```python
from build123d import *

# Parameters (mm, degrees)
SKETCH1_R               = 21
SKETCH1_R_2             = 16
BOSS_EXTRUDE1_DEPTH     = 10
SKETCH1_R_3             = 12.5
SKETCH1_R_4             = 6.25
BOSS_EXTRUDE1_2_DEPTH   = 10
BOSS_EXTRUDE2_DEPTH     = 6
CUT_EXTRUDE1_START      = -6
CUT_EXTRUDE1_DEPTH      = 22
CUT_EXTRUDE1_DEPTH_BACK = 16


with BuildPart() as part:
    # Sketch1 → Boss-Extrude1 (new body, symmetric)
    with BuildSketch(Plane.XY):
        Circle(SKETCH1_R)
        Circle(SKETCH1_R_2, mode=Mode.SUBTRACT)
    extrude(amount=BOSS_EXTRUDE1_DEPTH, both=True)



with BuildPart() as body_2:
    # Sketch1 → Boss-Extrude1 2 (new body, symmetric)
    with BuildSketch(Plane.XY):
        with Locations((0, 120)):
            Circle(SKETCH1_R_3)
        with Locations((0, 120)):
            Circle(SKETCH1_R_4, mode=Mode.SUBTRACT)
    extrude(amount=BOSS_EXTRUDE1_2_DEPTH, both=True)


with BuildPart() as part_1:
    add(part.part)

    add(body_2.part)  # Boss-Extrude2 merges body 2
    # Sketch1<4> → Boss-Extrude2 (add, symmetric)
    with BuildSketch(Plane.XY):
        with BuildLine():
            Line((-8, 110.395313644), (-8, 75.395313644))
            ThreePointArc((-8, 75.395313644), (-10.96842855, 40.709642053), (-19.787382488, 7.032744434))
            ThreePointArc((-19.787382488, 7.032744434), (0, 21), (19.787382488, 7.032744434))
            ThreePointArc((19.787382488, 7.032744434), (10.96842855, 40.709642053), (8, 75.395313644))
            Line((8, 75.395313644), (8, 110.395313644))
            ThreePointArc((8, 110.395313644), (0, 107.5), (-8, 110.395313644))
        make_face()
        with BuildLine():
            Line((-6.25, 135.825317547), (-6.25, 130.825317547))
            ThreePointArc((-6.25, 130.825317547), (0, 132.5), (6.25, 130.825317547))
            Line((6.25, 130.825317547), (6.25, 135.825317547))
            Line((6.25, 135.825317547), (-6.25, 135.825317547))
        make_face()
        with BuildLine():
            ThreePointArc((17, -12.328828006), (0, -21), (-17, -12.328828006))
            Line((-17, -12.328828006), (-17, -24.328828006))
            Line((-17, -24.328828006), (17, -24.328828006))
            Line((17, -24.328828006), (17, -12.328828006))
        make_face()
    extrude(amount=BOSS_EXTRUDE2_DEPTH, both=True)

    # Sketch2 → Cut-Extrude1 (cut, two sides)
    with BuildSketch(Plane(origin=(0, 0, 0), x_dir=(0, 0, -1), z_dir=(1, 0, 0)).offset(CUT_EXTRUDE1_START)) as cut_extrude1_sk:
        with BuildLine():
            Line((4, 100), (4, 38))
            ThreePointArc((4, 38), (0, 34), (-4, 38))
            Line((-4, 38), (-4, 100))
            ThreePointArc((-4, 100), (0, 104), (4, 100))
        make_face()
    extrude(amount=CUT_EXTRUDE1_DEPTH, mode=Mode.SUBTRACT)
    extrude(cut_extrude1_sk.sketch, amount=-CUT_EXTRUDE1_DEPTH_BACK, mode=Mode.SUBTRACT)


solid = part_1.part
```
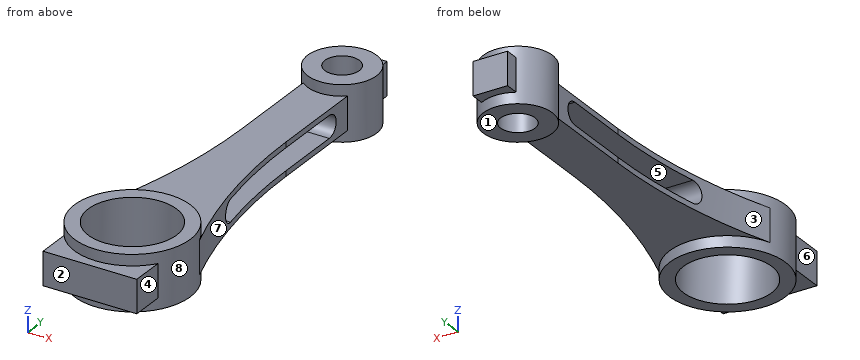
Input: part model. Units: mm. Frame: model coordinates. Face numbers are marked on the shaded views. A direction names the side the tool comes from. Round coordinates to 2 decimals unless told otherwise and drop trailing zeros. Write each loop counter-clockwise with the first axis right and the second up, starting at its lowest first coordinate (ties: lowest second). Pieces come first, ordered by that corner, then holes. Notation, with made-up numbers: (9, -30) - (59, -30) arc R14 ccw to (59, -15) - close; hole circle Ø10 at (85.5, 19). An arc over 180 degrees is marked (long way). Write item = value, one per line.
(1) Pull-direction query (Y, two-part tool) for the marked faces 1, 2 and 3; classes: +Y half, -Y half, draft (parallel to the pull), parting line (faces both ways), or undercut.
Geometry check:
face_1 = draft
face_2 = -Y half
face_3 = undercut
(2) Section query D-D on y = 120. Output: boundary loops of the cut face in (x, z), then the cut area to 3 significant figures.
Geometry check:
outline = (-12.5, -10) - (-6.25, -10) - (-6.25, 10) - (-12.5, 10) - close; (6.25, -10) - (12.5, -10) - (12.5, 10) - (6.25, 10) - close
area = 250 mm^2
(3) Section query C-C on y = 86.5. Output: boundary loops of the cut face in (x, z), then the cut area to 3 significant figures.
Geometry check:
outline = (-8, -6) - (8, -6) - (8, -4) - (-8, -4) - close; (-8, 4) - (8, 4) - (8, 6) - (-8, 6) - close
area = 64.0 mm^2
(4) Contact query for flat-ended pins moving along their axis: pin 1 Ø10 at (x, y) = (6, 94) entering from +Z; pin 2 Ø1 at (x, z) = (11.5, 5.5) entering from +Y; pin 3 Ø25 at (x, y) = (-2, 66) entering from -Z. Output: stop coordinate, or through.
Geometry check:
pin_1 = 6
pin_2 = 125.94
pin_3 = -6
(5) Section query B-B on z = 0. Output: boundary loops of the cut face in (x, y).
Geometry check:
outline = (-19.79, 7.03) arc R21 ccw to (-17, -12.33) - (-17, -24.33) - (17, -24.33) - (17, -12.33) arc R21 ccw to (19.79, 7.03) arc R204.13 cw to (12.24, 34) - (-12.24, 34) arc R204.13 cw to start; (-8, 104) - (8, 104) - (8, 110.4) arc R12.5 ccw to (6.25, 130.83) - (6.25, 135.83) - (-6.25, 135.83) - (-6.25, 130.83) arc R12.5 ccw to (-8, 110.4) - close; hole circle Ø32 at (0, 0); hole circle Ø12.5 at (0, 120)
(6) Section query A-A on x = 0. State how many separate pieces and enclosed holes the cut face has, then the cut area to 3 significant figures.
Geometry check:
separate_pieces = 3
enclosed_holes = 1
area = 1,020 mm^2
(7) Access query for the marked faces 4, 5, 6, 7 and 8. Directions: +Z, -Z, +X, -X, +Y, -Y. A direction counts if a zero-diameter tool reaches every point of the face in a straight line with its end or side. Return the directions, or none.
Geometry check:
face_4 = +Z, -Z, +X, -Y
face_5 = +X, -X
face_6 = +Z, -Z, -X, -Y
face_7 = +Z, -Z, +X
face_8 = none
(8) Material intervals for probe 1 along Y at (x, z) = (0, 5.75); probe 2 along Y at (x, z) = (-4, 7.75); probe 3 along Z at (x, y) = (-5.5, 86), sorted ascending.
Geometry check:
probe_1 = -24.33 to -16, 16 to 113.75, 126.25 to 135.83
probe_2 = -20.62 to -15.49, 15.49 to 20.62, 108.16 to 115.2, 124.8 to 131.84
probe_3 = -6 to -4, 4 to 6
